Study the drawing (mm; zero at the part's minimum x, y, z) and answer. A direction names the side the tool comes from. Round coordinates to 2 decimals unless told otherwise and drop trailing zeros. Order: outer loops, then holes, each group sorted by start corner. A loop starts at its lowest first (then second) coordinate and runs counter-clockwise, first axis right, second up. Notation, with made-up numbers: (-1.75, 43) - (32.25, 43) arc R13 ccw to (32.25, 55) - close; hole circle Ø10 at (4, 50.5). An arc over 180 degrees is marked (long way). Put each result on its own line as item: value. Start each with the question number.
Q1. For a pull along X with two mould halves and no side action, classify the marked faces 6, 7, 8 and 9 as pulls with the +X half, pulls with the -X half, needs draft (parallel to the pull), parting line crosses it, or undercut.
Q2. Section D-D on y = 30 is taken. Give the vertices of the cut face in (x, z), then the cut area to 3 significant figures.
Q3. Each of these flat-tipped pins is pushed along its axis until it touches: pin 1 Ø7 at (x, z) = (15, 9) entering from -Y; pin 2 Ø3 at (y, z) = (14, 8.5) entering from +X; pin 3 Ø5.5 at (y, z) = (7, 9.5) entering from -X. Where does it stop, or does it pass through?
Q4. Section B-B on z = 5.75 is taken. Give the vertices of the cut face in (x, y).
Q5. Find the intervals of material crossed by line 1 along Y through (x, z) = (25, 2); line 2 along X through (y, z) = (17.1, 9); line 3 along Z through (x, y) = (19, 3), in increasing order. Write a range as from..to.
Q6. Section C-C on z = 2 is taken. Give the vertices of the cut face in (x, y).
Q7. Section A-A on x = 5 is taken. Give the vertices of the cut face in (y, z), then the cut area to 3 significant figures.
Q8. Which of the six approach directions +Z, -Z, +X, -X, +Y, -Y give full straight-line access (tool end or side, diameter ignored) to the marked faces 1, 2, 3, 4 and 5?
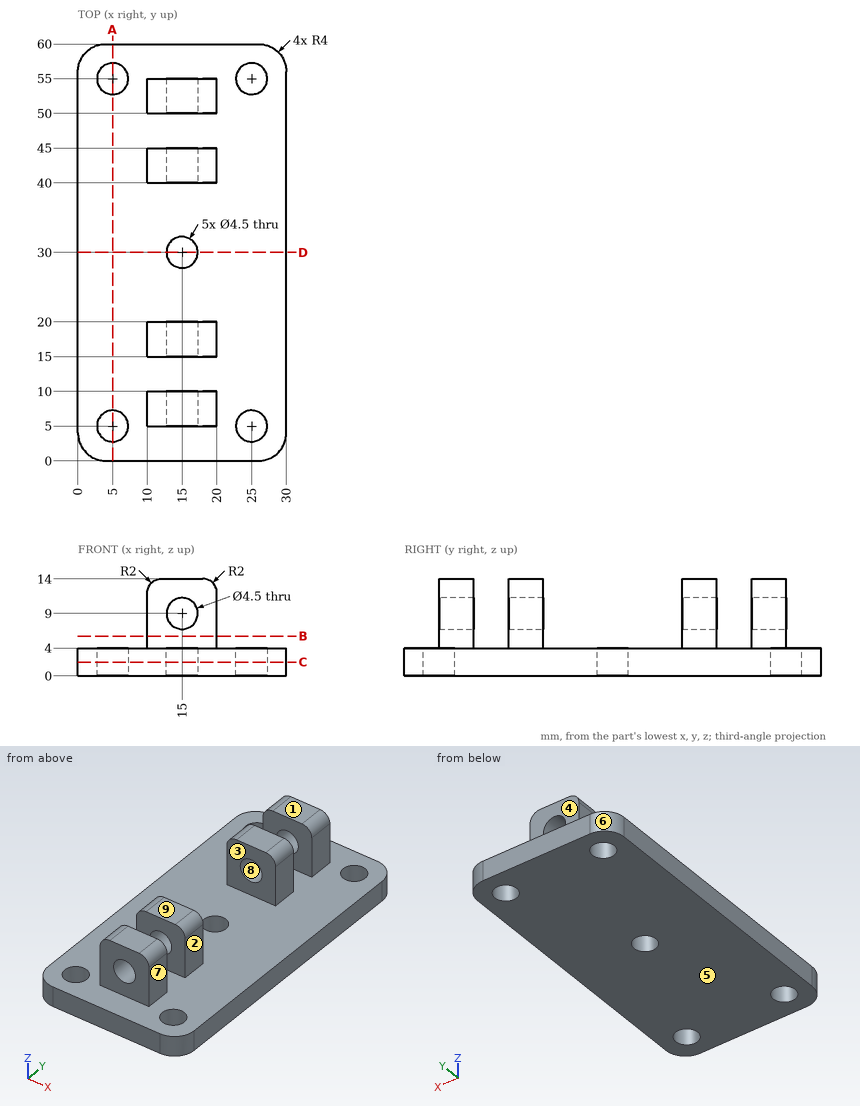
Findings:
1. face 6: pulls with the -X half
1. face 7: pulls with the +X half
1. face 8: undercut
1. face 9: needs draft
2. outline: (0, 0) - (12.75, 0) - (12.75, 4) - (0, 4) - close; (17.25, 0) - (30, 0) - (30, 4) - (17.25, 4) - close
2. area: 102 mm2
3. pin 1: y = 5
3. pin 2: x = 20
3. pin 3: x = 10
4. outline: (10, 5) - (20, 5) - (20, 10) - (10, 10) - close; (10, 15) - (20, 15) - (20, 20) - (10, 20) - close; (10, 40) - (20, 40) - (20, 45) - (10, 45) - close; (10, 50) - (20, 50) - (20, 55) - (10, 55) - close
5. line 1: 0..2.75, 7.25..52.75, 57.25..60
5. line 2: 10..12.75, 17.25..20
5. line 3: 0..4
6. outline: (0, 4) arc R4 ccw to (4, 0) - (26, 0) arc R4 ccw to (30, 4) - (30, 56) arc R4 ccw to (26, 60) - (4, 60) arc R4 ccw to (0, 56) - close; hole circle Ø4.5 at (5, 5); hole circle Ø4.5 at (5, 55); hole circle Ø4.5 at (15, 30); hole circle Ø4.5 at (25, 5); hole circle Ø4.5 at (25, 55)
7. outline: (0, 0) - (2.75, 0) - (2.75, 4) - (0, 4) - close; (7.25, 0) - (52.75, 0) - (52.75, 4) - (7.25, 4) - close; (57.25, 0) - (60, 0) - (60, 4) - (57.25, 4) - close
7. area: 204 mm2
8. face 1: +Z, +X, -X, +Y, -Y
8. face 2: +Z, +X, +Y, -Y
8. face 3: +Z, +X, -X
8. face 4: +Z, +X, -X, +Y
8. face 5: -Z, +X, -X, +Y, -Y
